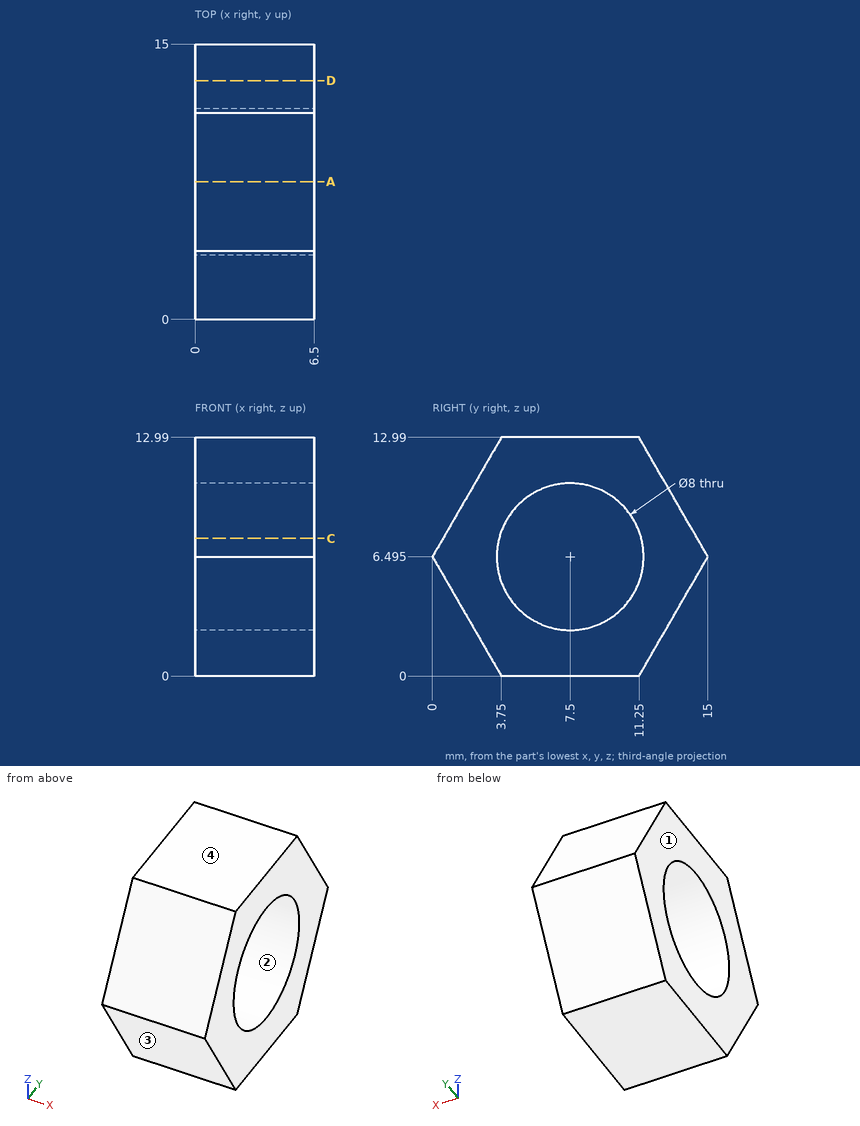
Input: dimensioned drawing with shaded views. Units: mm. Origin: part minimum x, y, z. Give positions to 0.01 mm unless a question says otherwise; leave off trailing zeros. Write each loop counter-clockwise with the first axis right and the second up, starting at its lowest first coordinate (ties: lowest second). Pieces come first, ordered by that corner, then holes. Notation, with made-up numbers: (74.5, 15) -> (117.5, 15) arc R18 ccw to (117.5, 27) -> close; hole circle Ø8 at (50.5, 23.25). An arc over 180 degrees is marked (long way). Return JSON: item names as keys, results as strings. Group by question number.
1. Section C-C, the plane z = 7.5. Output: boundary loops of the cut face in (x, y).
2. Material intervals for line 1 (Z direction, x = 2, y = 7.5) (1 decimal); line 2 (Y direction, x = 3, z = 4.75); line 3 (Y direction, x = 3, z = 8.5), sorted ascending. Write a range as from..to.
3. Section D-D, the plane y = 13. Output: boundary loops of the cut face in (x, z).
4. Section A-A, the plane y = 7.5. Output: boundary loops of the cut face in (x, z) (1 decimal).
5. Pin query (flat end, axial travel): pin 1 Ø1.5 at (x, z) = (2, 4) entering from -Y. Return the tip coordinate at first contact, or that it passes through.
6. Mould query, pull axis Z, two halves, no side actions, for the marked faces 1, 2, 3 and 4. Classes: +Z half, -Z half, draft (parallel to the pull), parting line (faces both ways), or undercut.
Determined:
{
 "1": {"outline": "(0, 0.58) -> (6.5, 0.58) -> (6.5, 3.63) -> (0, 3.63) -> close; (0, 11.37) -> (6.5, 11.37) -> (6.5, 14.42) -> (0, 14.42) -> close"},
 "2": {"line 1": "z = 0..2.5, 10.5..13", "line 2": "y = 1.01..3.9, 11.1..13.99", "line 3": "y = 1.16..4.04, 10.96..13.84"},
 "3": {"outline": "(0, 3.03) -> (6.5, 3.03) -> (6.5, 9.96) -> (0, 9.96) -> close"},
 "4": {"outline": "(0, 0) -> (6.5, 0) -> (6.5, 2.5) -> (0, 2.5) -> close; (0, 10.5) -> (6.5, 10.5) -> (6.5, 13) -> (0, 13) -> close"},
 "5": {"pin 1": "stops at y = 1.01"},
 "6": {"face 1": "draft", "face 2": "undercut", "face 3": "-Z half", "face 4": "+Z half"}
}
